Check sheet for the modelled part. Datum: model origin and axes. Units: mm. A direction names the side the tool comes from. Round coordinates to 2 decimals unless told otherwise and drop trailing zeros. Write each loop counter-clockwise with the first axis right and the second up, starting at its lowest first coordinate (ties: lowest second). Pieces come first, ordered by that corner, then holes.
Item 1: Section check B-B, the plane y = -1.5. Record the cut outline in (x, z).
Item 2: Set-up check for faces 3 (the flat face through (5.75, -10, 3)), 4 (the flat face through (-1, 1, 6.8)): record each of +Z, -Z, +X, -X, +Y, -Y from which the full face is reachable in a straight line by a thin tool's end or side.
Item 3: Section check C-C, the plane x = -23.25. Record the cut outline in (y, z), plus the area to 3 significant figures.
Item 4: Section check D-D, the plane x = -92. Record the cut outline in (y, z), plus the area to 3 significant figures.
Item 5: Release check for a two-part mould opening along Y. For faces 1 (the flat face through (-5.75, -10, 3)), 2 (the flat face through (-1, 1, 0)) record: pulls with the +Y half, pulls with the -Y half, needs draft (parallel to the pull), parting line crosses it, or undercut.
Item 6: Material ranges on line 1 along X through (y, z) = (9.5, 3); line 2 along Y through (x, z) = (23.25, 2.25); line 3 along Y through (x, z) = (0, 5), recorded low to high.
Item 7: Section check A-A, the plane x = 0. Record the cut outline in (y, z).
from build123d import *

# Parameters (mm, degrees)
SKETCH1_W            = 200
SKETCH1_H            = 84.3
BOSS_EXTRUDE1_DEPTH  = 6.8
SKETCH2_R            = 3.25
CUT_EXTRUDE1_DEPTH   = 6.8
FILLET1_R            = 2
SKETCH3_R            = 1.775
SKETCH3_W            = 42.5
SKETCH3_H            = 42.5
CUT_EXTRUDE2_DEPTH   = 7.8
FILLET2_R            = 2
SKETCH4_W            = 12
SKETCH4_H            = 7
CUT_EXTRUDE3_DEPTH   = 7.8
FILLET3_R            = 1.5
SKETCH5_R            = 1.75
SKETCH5_W            = 11.5
SKETCH5_H            = 12.5
CUT_EXTRUDE4_DEPTH   = 7.8
FILLET4_R            = 1.5
FILLET2_OF_MIRROR2_R = 2
FILLET3_OF_MIRROR2_R = 1.5


with BuildPart() as part:
    # Sketch1 → Boss-Extrude1 (new body)
    with BuildSketch(Plane.XY):
        Rectangle(SKETCH1_W, SKETCH1_H)
    extrude(amount=BOSS_EXTRUDE1_DEPTH)

    # Sketch2 → Cut-Extrude1 (cut)
    with BuildSketch(Plane.XY.offset(6.8)):
        with Locations((-92, 16.15)):
            Circle(SKETCH2_R)
        with Locations((92, 16.15)):
            Circle(SKETCH2_R)
    extrude(amount=-CUT_EXTRUDE1_DEPTH, mode=Mode.SUBTRACT)

    # Fillet1
    fillet1_edges = [part.edges().sort_by_distance(p)[0] for p in [
        (-100, 42.15, 3.4),
        (100, 42.15, 3.4),
        (100, -42.15, 3.4),
        (-100, -42.15, 3.4),
    ]]
    fillet(fillet1_edges, radius=FILLET1_R)

    # Sketch3 → Cut-Extrude2 (cut, through all)
    with BuildSketch(Plane.XY.offset(6.8)):
        with Locations((23.25, -26.082)):
            Circle(SKETCH3_R)
        with Locations((54.25, -26.082)):
            Circle(SKETCH3_R)
        with Locations((38.75, 10)):
            Rectangle(SKETCH3_W, SKETCH3_H)
    cut_extrude2 = extrude(amount=-CUT_EXTRUDE2_DEPTH, mode=Mode.SUBTRACT)

    # Fillet2
    fillet2_edges = [part.edges().sort_by_distance(p)[0] for p in [
        (17.5, -11.25, 3.4),
        (17.5, 31.25, 3.4),
        (60, 31.25, 3.4),
        (60, -11.25, 3.4),
    ]]
    fillet(fillet2_edges, radius=FILLET2_R)

    # Sketch4 → Cut-Extrude3 (cut, through all)
    with BuildSketch(Plane.XY.offset(6.8)):
        with Locations((38.75, -11.25)):
            Rectangle(SKETCH4_W, SKETCH4_H)
    cut_extrude3 = extrude(amount=-CUT_EXTRUDE3_DEPTH, mode=Mode.SUBTRACT)

    # Fillet3
    fillet3_edges = [part.edges().sort_by_distance(p)[0] for p in [
        (44.75, -11.25, 3.4),
        (32.75, -11.25, 3.4),
        (32.75, -14.75, 3.4),
        (44.75, -14.75, 3.4),
    ]]
    fillet(fillet3_edges, radius=FILLET3_R)

    # Sketch5 → Cut-Extrude4 (cut, through all)
    with BuildSketch(Plane.XY.offset(6.8)):
        with Locations((0, -25)):
            Circle(SKETCH5_R)
        with Locations((0, 5)):
            Circle(SKETCH5_R)
        with Locations((0, -10)):
            Rectangle(SKETCH5_W, SKETCH5_H)
    extrude(amount=-CUT_EXTRUDE4_DEPTH, mode=Mode.SUBTRACT)

    # Fillet4
    fillet4_edges = [part.edges().sort_by_distance(p)[0] for p in [
        (-5.75, -16.25, 3.4),
        (-5.75, -3.75, 3.4),
        (5.75, -3.75, 3.4),
        (5.75, -16.25, 3.4),
    ]]
    fillet(fillet4_edges, radius=FILLET4_R)

    # Mirror2: Cut-Extrude2, Cut-Extrude3 across plane
    add(cut_extrude2.mirror(Plane(origin=(0, 0, 0), x_dir=(0, 0, 1), z_dir=(1, 0, 0))), mode=Mode.SUBTRACT)
    add(cut_extrude3.mirror(Plane(origin=(0, 0, 0), x_dir=(0, 0, 1), z_dir=(1, 0, 0))), mode=Mode.SUBTRACT)

    # Fillet2 of Mirror2
    fillet2_of_mirror2_edges = [part.edges().sort_by_distance(p)[0] for p in [
        (-17.5, -11.25, 3.4),
        (-17.5, 31.25, 3.4),
        (-60, 31.25, 3.4),
        (-60, -11.25, 3.4),
    ]]
    fillet(fillet2_of_mirror2_edges, radius=FILLET2_OF_MIRROR2_R)

    # Fillet3 of Mirror2
    fillet3_of_mirror2_edges = [part.edges().sort_by_distance(p)[0] for p in [
        (-44.75, -11.25, 3.4),
        (-32.75, -11.25, 3.4),
        (-32.75, -14.75, 3.4),
        (-44.75, -14.75, 3.4),
    ]]
    fillet(fillet3_of_mirror2_edges, radius=FILLET3_OF_MIRROR2_R)


solid = part.part
Values found:
1. outline: (-100, 0) - (-60, 0) - (-60, 6.8) - (-100, 6.8) - close; (-17.5, 0) - (17.5, 0) - (17.5, 6.8) - (-17.5, 6.8) - close; (60, 0) - (100, 0) - (100, 6.8) - (60, 6.8) - close
2. face 3: +Z, -Z
2. face 4: +Z, +X, -X, +Y, -Y
3. outline: (-42.15, 0) - (-27.86, 0) - (-27.86, 6.8) - (-42.15, 6.8) - close; (-24.31, 0) - (-11.25, 0) - (-11.25, 6.8) - (-24.31, 6.8) - close; (31.25, 0) - (42.15, 0) - (42.15, 6.8) - (31.25, 6.8) - close
3. area: 260 mm2
4. outline: (-42.15, 0) - (12.9, 0) - (12.9, 6.8) - (-42.15, 6.8) - close; (19.4, 0) - (42.15, 0) - (42.15, 6.8) - (19.4, 6.8) - close
4. area: 529 mm2
5. face 1: undercut
5. face 2: needs draft
6. line 1: x = -100 to -60, -17.5 to 17.5, 60 to 100
6. line 2: y = -42.15 to -27.86, -24.31 to -11.25, 31.25 to 42.15
6. line 3: y = -42.15 to -26.75, -23.25 to -16.25, -3.75 to 3.25, 6.75 to 42.15
7. outline: (-42.15, 0) - (-26.75, 0) - (-26.75, 6.8) - (-42.15, 6.8) - close; (-23.25, 0) - (-16.25, 0) - (-16.25, 6.8) - (-23.25, 6.8) - close; (-3.75, 0) - (3.25, 0) - (3.25, 6.8) - (-3.75, 6.8) - close; (6.75, 0) - (42.15, 0) - (42.15, 6.8) - (6.75, 6.8) - close
